The model under review builds one solid part; all positions refer to its coordinate system, in mm. Face numbers are marked on the shaded views. A direction names the side the tool comes from. Round coordinates to 2 decimals unless told otherwise and drop trailing zeros. Write each loop counter-clockwise with the first axis right and the second up, starting at its lowest first coordinate (ties: lowest second). Pieces come first, ordered by that corner, then holes. Notation, with made-up numbers: (-9.75, -34.5) -> (39.25, -34.5) arc R7 ccw to (39.25, -28.5) -> close; hole circle Ø8 at (49.5, 85). An arc over 180 degrees is marked (long way). Return JSON: item names as keys, results as strings. Group by question number.
1. For line 1 along X through (y, z) = (11, 9); line 2 along Y through (x, z) = (38, 18); line 3 along Z through (x, y) = (36.5, 15), list the stretches that pass through material, from the lowest coordinate up. Write a range as from..to.
2. Tool access review of the marked faces 1 and 2: name each direction out of +Z, -Z, +X, -X, +Y, -Y from which nothing blocks a thin tool from reaching the whole face with its end or side.
3. Take a section at A-A, the plane z = 0. Write out the cut boundary in (x, y).
4. Clearance check with a flat-ended pin moving along its axis: P1, Ø6, axis at x = 40.5, y = 12, coming from the +Z side. State where the tip first meets the part, or that it passes through.
5. Take a section at B-B, the plane y = 16.25. Write out the cut boundary in (x, z).
6. Take a section at C-C, the plane z = -9. Write out the cut boundary in (x, y).
7. Take a section at D-D, the plane y = 10. Write out the cut boundary in (x, z), then the cut area to 3 significant figures.
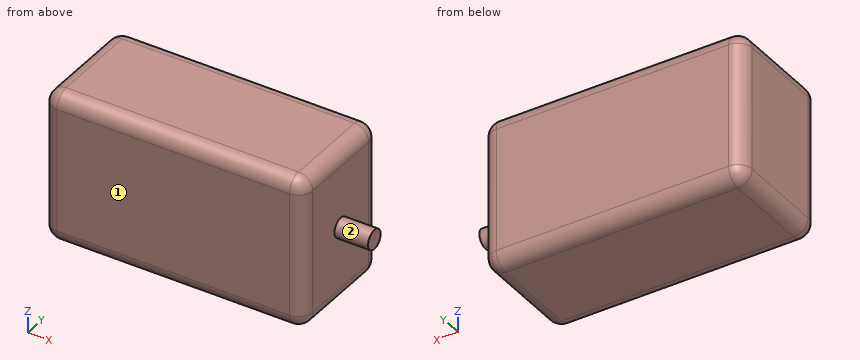
from build123d import *

# Parameters (mm, degrees)
SKETCH1_W           = 73.6
SKETCH1_H           = 42.8
BOSS_EXTRUDE1_DEPTH = 32.5
SKETCH2_R           = 2.75
BOSS_EXTRUDE2_DEPTH = 9.5
FILLET1_R           = 4


with BuildPart() as part:
    # Sketch1 → Boss-Extrude1 (new body)
    with BuildSketch(Plane(origin=(0, 0, 0), x_dir=(1, 0, 0), z_dir=(0, 1, 0))):
        with Locations((3.258713578, 0)):
            Rectangle(SKETCH1_W, SKETCH1_H)
    extrude(amount=BOSS_EXTRUDE1_DEPTH)

    # Sketch2 → Boss-Extrude2 (add)
    with BuildSketch(Plane(origin=(40.058713578, 0, 0), x_dir=(0, 0, -1), z_dir=(1, 0, 0))):
        with Locations((0, 16.25)):
            Circle(SKETCH2_R)
    extrude(amount=BOSS_EXTRUDE2_DEPTH)

    # Fillet1
    fillet1_edges = [part.edges().sort_by_distance(p)[0] for p in [
        (-33.541286422, 32.5, 0),
        (3.258713578, 32.5, 21.4),
        (40.058713578, 32.5, 0),
        (3.258713578, 0, 21.4),
        (-33.541286422, 0, 0),
        (3.258713578, 0, -21.4),
        (40.058713578, 0, 0),
        (40.058713578, 16.25, 21.4),
        (-33.541286422, 16.25, 21.4),
        (-33.541286422, 16.25, -21.4),
        (40.058713578, 16.25, -21.4),
        (3.258713578, 32.5, -21.4),
    ]]
    fillet(fillet1_edges, radius=FILLET1_R)


solid = part.part
Output:
{
 "1": {"line 1": "x = -33.54..40.06", "line 2": "y = 0.55..31.95", "line 3": "z = -21.38..21.38"},
 "2": {"face 1": "+Z, -Z, +X, -X, -Y", "face 2": "+X"},
 "3": {"outline": "(-33.54, 4) arc R4 ccw to (-29.54, 0) -> (36.06, 0) arc R4 ccw to (40.06, 4) -> (40.06, 13.5) -> (49.56, 13.5) -> (49.56, 19) -> (40.06, 19) -> (40.06, 28.5) arc R4 ccw to (36.06, 32.5) -> (-29.54, 32.5) arc R4 ccw to (-33.54, 28.5) -> close"},
 "4": {"P1": "stops at z = 21.13"},
 "5": {"outline": "(-33.54, -17.4) arc R4 ccw to (-29.54, -21.4) -> (36.06, -21.4) arc R4 ccw to (40.06, -17.4) -> (40.06, -2.75) -> (49.56, -2.75) -> (49.56, 2.75) -> (40.06, 2.75) -> (40.06, 17.4) arc R4 ccw to (36.06, 21.4) -> (-29.54, 21.4) arc R4 ccw to (-33.54, 17.4) -> close"},
 "6": {"outline": "(-33.54, 4) arc R4 ccw to (-29.54, 0) -> (36.06, 0) arc R4 ccw to (40.06, 4) -> (40.06, 28.5) arc R4 ccw to (36.06, 32.5) -> (-29.54, 32.5) arc R4 ccw to (-33.54, 28.5) -> close"},
 "7": {"outline": "(-33.54, -17.4) arc R4 ccw to (-29.54, -21.4) -> (36.06, -21.4) arc R4 ccw to (40.06, -17.4) -> (40.06, 17.4) arc R4 ccw to (36.06, 21.4) -> (-29.54, 21.4) arc R4 ccw to (-33.54, 17.4) -> close", "area": "3,140 mm^2"}
}
